Autodesk Inventor part; units mm, degrees
ref_plane "YZ Plane" through (0, 0, 0) normal (1, 0, 0) x (0, 1, 0)
ref_plane "XZ Plane" through (0, 0, 0) normal (0, 1, 0) x (-1, 0, 0)
ref_plane "XY Plane" through (0, 0, 0) normal (0, 0, 1) x (1, 0, 0)
sketch "Sketch1" plane through (0, 0, 0) normal (0, 1, 0) x (-1, 0, 0)
  line L0 (-13.5, 13.5) -> (13.5, 13.5)
  line L1 (13.5, 13.5) -> (13.5, -13.5)
  line L2 (13.5, -13.5) -> (-13.5, -13.5)
  line L3 (-13.5, -13.5) -> (-13.5, 13.5)
  line L4 (-13.5, 13.5) -> (13.5, -13.5) construction
  line L5 (13.5, 13.5) -> (-13.5, -13.5) construction
  line L6 (11.5, -11.5) -> (11.5, 11.5)
  line L7 (11.5, 11.5) -> (-11.5, 11.5)
  line L8 (-11.5, 11.5) -> (-11.5, -11.5)
  line L9 (-11.5, -11.5) -> (11.5, -11.5)
  line L10 (11.5, 11.5) -> (13.5, 11.5)
  line L11 (11.5, -11.5) -> (13.5, -11.5)
  point P0 (0, 0)
  dimension "d0" = 27
  dimension "d1" = 27
  dimension "d2" = 2
extrude "Extrusion1" add sketch "Sketch1" along normal blind 279.4 contours L0 L1 L10 L7 L8 L9 L11 L2 L3
sketch "Sketch2" plane through (-13.5, 0, 13.5) normal (0, 0, 1) x (1, 0, 0)
  line L0 (13.5, 0) -> (13.5, 12.7) construction
  circle A0 centre (13.5, 12.7) radius 4
  dimension "d5" = 12.7
  dimension "d6" = 8
sketch "Sketch3" plane through (13.5, 0, 13.5) normal (1, 0, 0) x (0, 0, -1)
  line L0 (13.5, 0) -> (13.5, 12.7) construction
  circle A0 centre (13.5, 12.7) radius 4
  dimension "d7" = 12.7
  dimension "d8" = 8
extrude "Extrusion2" cut sketch "Sketch2" against normal blind 93.1875
extrude "Extrusion3" cut sketch "Sketch3" against normal blind 117.95
pattern_linear "Rectangular Pattern1" count 11 spacing 25.4 along (0, 1, 0) of "Extrusion2", "Extrusion3"
properties part number "C-Channel 11in" material "Aluminum 6061"
Source: CAD feature listing. Evaluate the final solid. Frame: model axes, mm. A direction names the side the tool comes from. Coordinates: 2 decimals unless noted, no trailing zeros. Write each loop counter-clockwise with the first axis right and the second up, starting at its lowest first coordinate (ties: lowest second). Pieces come first, ordered by that corner, then holes. Notation, with made-up numbers: M -4,58.25 L 21,58.25 A23 ccw 21,68.25 Z; hole C 79.5,-5 d8. An arc over 180 degrees is marked long. Answer as a JSON object with one key per item and string values.
1. Contact query for a flat-ended pin moving along its axis: P1, Ø1, axis at y = 61, z = 5.5, coming from the -X side. Output: stop coordinate, or through.
Evaluation:
{"P1": "x = 11.5"}
2. Cut plane B-B on x = -11. Output: boundary loops of the cut face in (y, z), plus the area to 3 significant figures.
Evaluation:
{"outline": "M 0,-13.5 L 279.4,-13.5 L 279.4,-11.5 L 0,-11.5 Z; M 0,11.5 L 279.4,11.5 L 279.4,13.5 L 0,13.5 Z", "area": "1,120 mm^2"}
3. Access query for faces 4 (the cylindrical face through (1.846, 263.151, -12.486)), 5 (the flat face through (-4, 138, -11.5)). Directions: +Z, -Z, +X, -X, +Y, -Y. A direction counts if a zero-diameter tool reaches every point of the face in a straight line with its end or side. Return the directions, or none.
Evaluation:
{"face 4": "+Z, -Z", "face 5": "-X, +Y, -Y"}
4. Draft query along Z for faces 1 (the cylindrical face through (-0.521, 219.866, -12.486)), 2 (the flat face through (-6, 138, -13.5)), 3 (the cylindrical face through (12.514, 263.151, -1.846)). Return one class per face: released by +Z, released by -Z, zero draft, split by the parting line, or undercut.
Evaluation:
{"face 1": "zero draft", "face 2": "released by -Z", "face 3": "undercut"}
5. Cut plane C-C on y = 30. Output: boundary loops of the cut face in (x, z).
Evaluation:
{"outline": "M -13.5,-13.5 L 13.5,-13.5 L 13.5,13.5 L -13.5,13.5 L -13.5,11.5 L 11.5,11.5 L 11.5,-11.5 L -13.5,-11.5 Z"}
6. Cut plane D-D on x = 0. State how many separate pieces and enclosed holes the cut face has, plus the area to 3 significant figures.
Evaluation:
{"separate pieces": "24", "enclosed holes": "0", "area": "766 mm^2"}
7. Ray query, L1, parallel to Z at x = 4, y = 224.5; L2, parallel to X at y = 62.5, z = 5.25; L3, parallel to Z at x = 12.6, y = 266.7. Return the intervals inside material, ascending.
Evaluation:
{"L1": "-13.5 to -11.5, 11.5 to 13.5", "L2": "11.5 to 13.5", "L3": "-13.5 to -4, 4 to 13.5"}
8. Cut plane A-A on y = 88.9. Output: boundary loops of the cut face in (x, z).
Evaluation:
{"outline": "M -13.5,-13.5 L -4,-13.5 L -4,-11.5 L -13.5,-11.5 Z; M -13.5,11.5 L -4,11.5 L -4,13.5 L -13.5,13.5 Z; M 4,-13.5 L 13.5,-13.5 L 13.5,-4 L 11.5,-4 L 11.5,-11.5 L 4,-11.5 Z; M 4,11.5 L 11.5,11.5 L 11.5,4 L 13.5,4 L 13.5,13.5 L 4,13.5 Z"}
